```python
from build123d import *

# Parameters (mm, degrees)
POCKET_DEPTH       = 16
POLARPATTERN_COUNT = 6


with BuildPart() as part:
    # Sketch → Revolution (revolve)
    with BuildSketch(Plane.XY):
        Polygon((-12, 15), (12, 15), (12, 22.5), (8, 22.5), (8, 70), (27.155, 90), (27.155, 115), (25.905, 115), (19.352321, 97), (16.852321, 97), (10.300857, 115), (7.800857, 115), (1.249393, 97), (-1.250607, 97), (-7.802072, 115), (-10.302072, 115), (-16.853536, 97), (-19.353536, 97), (-25.905, 115), (-27.155, 115), (-27.155, 90), (-8, 70), (-8, 22.5), (-12, 22.5), align=None)
    revolve(axis=Axis((0, 0, 0), (1, 0, 0)))

    # Sketch001 (on Face7 of Revolution) → Pocket (cut)
    with BuildSketch(Plane.YZ.offset(8)):
        with BuildLine():
            ThreePointArc((5.823465, 21.733321), (0, 22.5), (-5.823465, 21.733321))
            Line((-18.11737, 67.614798), (-5.823465, 21.733321))
            ThreePointArc((18.11737, 67.614798), (0, 70), (-18.11737, 67.614798))
            Line((18.11737, 67.614798), (5.823465, 21.733321))
        make_face()
    pocket = extrude(amount=-POCKET_DEPTH, mode=Mode.SUBTRACT)

    # PolarPattern: Pocket ×6 about axis
    polarpattern_axis = Axis((8, 0, 0), (1, 0, 0))
    for i in range(1, POLARPATTERN_COUNT):
        add(pocket.rotate(polarpattern_axis, i * 360 / POLARPATTERN_COUNT), mode=Mode.SUBTRACT)


solid = part.part
```
Read the model definition and answer for the solid it produces. Units are mm, in the model's axes. A direction names the side the tool comes from. Coordinates: 2 decimals unless noted, no trailing zeros. Answer as a JSON object with one key per item and string values.
Q1. Consider line 1 (X direction, y = 43.5, z = -105) (3 decimals); line 2 (X direction, y = -0.5, z = -104) (3 decimals); line 3 (X direction, y = -67.5, z = 18). Determine where each line is inside the solid, lowest interval first. Write a range as [from, to].
The answers:
{"line 1": "x = [-27.155, -25.415], [-10.792, -7.312], [7.311, 10.791], [25.415, 27.155]", "line 2": "x = [-27.155, -21.902], [-14.305, -3.799], [3.798, 14.304], [21.901, 27.155]", "line 3": "x = [-8, 8]"}
Q2. The part is cut by section A-A on y = 0. Give the number of separate pieces and of enclosed holes in the cut face, then the cut area to 3 significant figures.
The answers:
{"separate pieces": "4", "enclosed holes": "0", "area": "3,500 mm2"}
Q3. Flat-ended cylindrical pins translate along their axes: pin 1 Ø13 at (y, z) = (-35, -30.5) entering from +X; pin 2 Ø22 at (y, z) = (-24.5, -48) entering from -X; pin 3 Ø1.5 at (y, z) = (30, -63.5) entering from +X. Find the tip coordinate at first contact, or state that the pin passes through.
The answers:
{"pin 1": "stops at x = 8", "pin 2": "stops at x = -8", "pin 3": "stops at x = 8.94"}
Q4. A tool of negligible diameter and unlimited length cuts with its end or side. For faces 3 (the conical face through (-16.535, 93.354, 29.399)), 4 (the flat face through (8, 23, -41)), 5 (the flat face through (0.112, -44.995, 12.056)), 6 (the flat face through (-12, 15, -5)), from which of +Z, -Z, +X, -X, +Y, -Y can it reach the whole face along a straight path? Write none if from no direction.
The answers:
{"face 3": "none", "face 4": "+X", "face 5": "+X, -X", "face 6": "-X"}
Q5. Determine the mould class of faces 1 (the conical face through (-8.93, 65.56, -27.18)), 2 (the conical face through (-19.763, -21.272, -95.793)) for opening direction Z: pulls with the +Z half, pulls with the -Z half, needs draft (parallel to the pull), parting line crosses it, or undercut.
The answers:
{"face 1": "undercut", "face 2": "parting line crosses it"}
